Model file for the job. Use its own axes, mm. Round coordinates to 2 decimals unless told otherwise and drop trailing zeros. Loops run counter-clockwise (first coordinate to the right, second up) from the corner with the lowest first, then second, coordinate; pieces in that order, holes last. Notation, with made-up numbers: (-22.75, 83) - (-18.75, 83) arc R20 ccw to (-18.75, 96) - close; hole circle Ø7 at (-22, 75). An arc over 180 degrees is marked (long way). Use one line per item in the form item = value.
from build123d import *

# Parameters (mm, degrees)
SKETCH1_R           = 6.35
SKETCH1_R_2         = 1.5875
SKETCH1_W           = 127
SKETCH1_H           = 127
BOSS_EXTRUDE1_DEPTH = 2.54


with BuildPart() as part:
    # Sketch1 → Boss-Extrude1 (new body)
    with BuildSketch(Plane.XY):
        Polygon((141.2875, 192.0875), (-141.2875, 192.0875), (-141.2875, -192.0875), (-15.008193375, -192.0875), (-15.008193375, -93.6625), (16.741806625, -93.6625), (16.741806625, -192.0875), (141.2875, -192.0875), align=None)
        with Locations((-128.5875, -169.8625)):
            Circle(SKETCH1_R, mode=Mode.SUBTRACT)
        with Locations((-128.5875, -1.5875)):
            Circle(SKETCH1_R, mode=Mode.SUBTRACT)
        with Locations((-80.175152311, -5.023613243)):
            Circle(SKETCH1_R_2, mode=Mode.SUBTRACT)
        with Locations((128.5875, -169.8625)):
            Circle(SKETCH1_R, mode=Mode.SUBTRACT)
        with Locations((79.970650499, -5.395164494)):
            Circle(SKETCH1_R_2, mode=Mode.SUBTRACT)
        with Locations((128.5875, -1.5875)):
            Circle(SKETCH1_R, mode=Mode.SUBTRACT)
        with Locations((-80.175152311, 71.176386757)):
            Circle(SKETCH1_R_2, mode=Mode.SUBTRACT)
        with Locations((-0.006402311, 49.2125)):
            Rectangle(SKETCH1_W, SKETCH1_H, mode=Mode.SUBTRACT)
        with Locations((-128.5875, 166.6875)):
            Circle(SKETCH1_R, mode=Mode.SUBTRACT)
        with Locations((-80.175152311, 147.376386757)):
            Circle(SKETCH1_R_2, mode=Mode.SUBTRACT)
        with Locations((79.970650499, 70.804835506)):
            Circle(SKETCH1_R_2, mode=Mode.SUBTRACT)
        with Locations((79.970650499, 147.004835506)):
            Circle(SKETCH1_R_2, mode=Mode.SUBTRACT)
        with Locations((128.5875, 166.6875)):
            Circle(SKETCH1_R, mode=Mode.SUBTRACT)
    extrude(amount=BOSS_EXTRUDE1_DEPTH)


solid = part.part
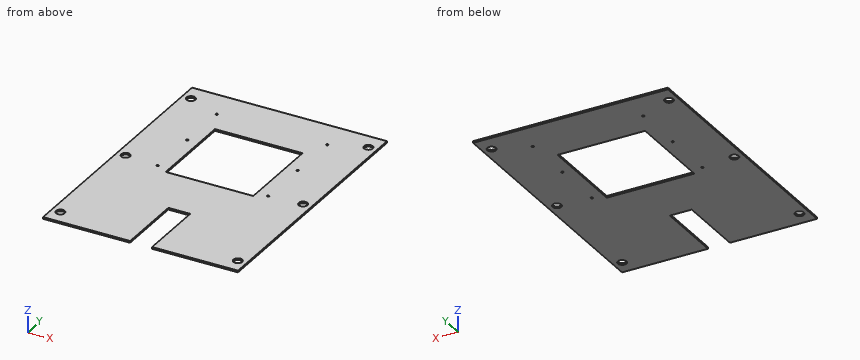
1. Cut at B-B, the plane y = 103. Give the cut face in (x, z), plus the area to 3 significant figures.
Geometry check:
outline = (-141.29, 0) - (-63.51, 0) - (-63.51, 2.54) - (-141.29, 2.54) - close; (63.49, 0) - (141.29, 0) - (141.29, 2.54) - (63.49, 2.54) - close
area = 395 mm^2
2. Flat gauge pins, fed straight in: pin 1 (1.3 mm diameter, centred on x = -3.5, z = 1.5, fed in from -Y); pin 2 (2.5 mm diameter, centred on x = -80.18, y = 71.18, fed in from -Z). Where does each tip first touch, or does it go through?
Geometry check:
pin_1 = -93.66
pin_2 = through
3. Cut at A-A, the plane x = 36. Give the cut face in (y, z), plus the area to 3 significant figures.
Geometry check:
outline = (-192.09, 0) - (-14.29, 0) - (-14.29, 2.54) - (-192.09, 2.54) - close; (112.71, 0) - (192.09, 0) - (192.09, 2.54) - (112.71, 2.54) - close
area = 653 mm^2
4. Cut at C-C, the plane z = 1.3. Give the number of separate pieces and of enclosed holes in the cut face, plus the area to 3 significant figures.
Geometry check:
separate_pieces = 1
enclosed_holes = 13
area = 88,500 mm^2
5. Wall check: probe 1 along X at (y, z) = (53.5, 2.1); probe 2 along Y at (x, z) = (-43, 2); probe 3 along X at (y, z) = (-152.5, 1.75). Give the ranges that are in metal, low to high.
Geometry check:
probe_1 = -141.29 to -63.51, 63.49 to 141.29
probe_2 = -192.09 to -14.29, 112.71 to 192.09
probe_3 = -141.29 to -15.01, 16.74 to 141.29
